Build history of the part. All positions in model axes, mm. A direction names the side the tool comes from. Round coordinates to 2 decimals unless told otherwise and drop trailing zeros. Write each loop counter-clockwise with the first axis right and the second up, starting at its lowest first coordinate (ties: lowest second). Pieces come first, ordered by that corner, then holes.
Item 1: 3-axis set-ups, long thin cutter, end or side, ignore diameter. For faces 1 (the flat face through (-23, 42.483, 3)), 2 (the flat face through (21.963, 47, 3)), 3 (the flat face through (37, 9.483, 3)): which of +Z, -Z, +X, -X, +Y, -Y reach the whole face in a straight line?
Item 2: Band-saw the part on B-B, the plane x = -21. Write the cut outline in (y, z), then the cut area to 3 significant figures.
Item 3: Wall check: probe 1 along X at (y, z) = (14.5, 2.5); probe 2 along Y at (x, z) = (2.5, 5); probe 3 along X at (y, z) = (-18, 0.5). Give the ranges that are in metal, low to high.
Item 4: Band-saw the part on D-D, the plane z = 2.5. Count the separate pieces of the cut face and the enclosed holes in it, then the cut area to 3 significant figures.
Item 5: Drop flat-ended pins along their axis: pin 1 Ø1.8 at (x, z) = (36.5, 2) entering from +Y; pin 2 Ø1 at (x, z) = (33, 2) entering from -Y; pin 3 Ø1.5 at (y, z) = (-8.5, 5.5) entering from +X. Give the stop position or say it passes through.
Item 6: Mould opens along Y. For faces 4 (the flat face through (27, -25.517, 3)), 5 (the cylindrical face through (21.393, 51.882, 3.131)), 6 (the cylindrical face through (7.86, 9.5, 3.22)) say: +Y half, -Y half, draft (parallel to the pull), parting line (faces both ways), or undercut.
Item 7: Band-saw the part on C-C, the plane y = -21. Write the cut outline in (x, z), then the cut area to 3 significant figures.
Item 8: Band-saw the part on A-A, the plane x = -5.5. Write the cut outline in (y, z).
```python
from build123d import *

# Parameters (mm, degrees)
EXTRUDE_1_DEPTH     = 6.35
SKETCH_2_R          = 1.5
CUT_EXTRUDE_1_DEPTH = 7.35
SKETCH_3_R          = 3
SKETCH_3_R_2        = 1.5
CUT_EXTRUDE_2_DEPTH = 7.35


with BuildPart() as part:
    # 草图1 → 凸台-拉伸1 (new body)
    with BuildSketch(Plane.XY):
        with BuildLine():
            Line((-28.036772487, 40.483201058), (-28.036772487, 21.483201058))
            ThreePointArc((-28.036772487, 21.483201058), (-28.622558924, 20.068987496), (-30.036772487, 19.483201058))
            Line((-30.036772487, 19.483201058), (-36.036772487, 19.483201058))
            ThreePointArc((-36.036772487, 19.483201058), (-37.450986049, 18.897414621), (-38.036772487, 17.483201058))
            Line((-38.036772487, 17.483201058), (-38.036772487, 11.483201058))
            ThreePointArc((-38.036772487, 11.483201058), (-37.450986049, 10.068987496), (-36.036772487, 9.483201058))
            Line((-36.036772487, 9.483201058), (-30.036772487, 9.483201058))
            ThreePointArc((-30.036772487, 9.483201058), (-28.622558924, 8.897414621), (-28.036772487, 7.483201058))
            Line((-28.036772487, 7.483201058), (-28.036772487, -23.516798942))
            ThreePointArc((-28.036772487, -23.516798942), (-27.450986049, -24.931012504), (-26.036772487, -25.516798942))
            Line((-26.036772487, -25.516798942), (-20.036772487, -25.516798942))
            ThreePointArc((-20.036772487, -25.516798942), (-18.622558924, -26.102585379), (-18.036772487, -27.516798942))
            Line((-18.036772487, -27.516798942), (-18.036772487, -33.516798942))
            ThreePointArc((-18.036772487, -33.516798942), (-17.450986049, -34.931012504), (-16.036772487, -35.516798942))
            Line((-16.036772487, -35.516798942), (19.963227513, -35.516798942))
            ThreePointArc((19.963227513, -35.516798942), (21.377441076, -34.931012504), (21.963227513, -33.516798942))
            Line((21.963227513, -33.516798942), (21.963227513, -27.516798942))
            ThreePointArc((21.963227513, -27.516798942), (22.549013951, -26.102585379), (23.963227513, -25.516798942))
            Line((23.963227513, -25.516798942), (29.963227513, -25.516798942))
            ThreePointArc((29.963227513, -25.516798942), (31.377441076, -24.931012504), (31.963227513, -23.516798942))
            Line((31.963227513, -23.516798942), (31.963227513, 7.483201058))
            ThreePointArc((31.963227513, 7.483201058), (32.549013951, 8.897414621), (33.963227513, 9.483201058))
            Line((33.963227513, 9.483201058), (39.963227513, 9.483201058))
            ThreePointArc((39.963227513, 9.483201058), (41.377441076, 10.068987496), (41.963227513, 11.483201058))
            Line((41.963227513, 11.483201058), (41.963227513, 17.483201058))
            ThreePointArc((41.963227513, 17.483201058), (41.377441076, 18.897414621), (39.963227513, 19.483201058))
            Line((39.963227513, 19.483201058), (33.963227513, 19.483201058))
            ThreePointArc((33.963227513, 19.483201058), (32.549013951, 20.068987496), (31.963227513, 21.483201058))
            Line((31.963227513, 21.483201058), (31.963227513, 40.483201058))
            ThreePointArc((31.963227513, 40.483201058), (31.377441076, 41.897414621), (29.963227513, 42.483201058))
            Line((29.963227513, 42.483201058), (23.963227513, 42.483201058))
            ThreePointArc((23.963227513, 42.483201058), (22.549013951, 43.068987496), (21.963227513, 44.483201058))
            Line((21.963227513, 44.483201058), (21.963227513, 50.483201058))
            ThreePointArc((21.963227513, 50.483201058), (21.377441076, 51.897414621), (19.963227513, 52.483201058))
            Line((19.963227513, 52.483201058), (-16.036772487, 52.483201058))
            ThreePointArc((-16.036772487, 52.483201058), (-17.450986049, 51.897414621), (-18.036772487, 50.483201058))
            Line((-18.036772487, 50.483201058), (-18.036772487, 44.483201058))
            ThreePointArc((-18.036772487, 44.483201058), (-18.622558924, 43.068987496), (-20.036772487, 42.483201058))
            Line((-20.036772487, 42.483201058), (-26.036772487, 42.483201058))
            ThreePointArc((-26.036772487, 42.483201058), (-27.450986049, 41.897414621), (-28.036772487, 40.483201058))
        make_face()
    extrude(amount=EXTRUDE_1_DEPTH)

    # 草图2 → 切除-拉伸1 (cut, through all)
    with BuildSketch(Plane.XY.offset(6.35)):
        with Locations((-33.036772487, 14.483201058)):
            Circle(SKETCH_2_R)
        with Locations((36.963227513, 14.483201058)):
            Circle(SKETCH_2_R)
    extrude(amount=-CUT_EXTRUDE_1_DEPTH, mode=Mode.SUBTRACT)

    # 草图3 → 切除-拉伸2 (cut, through all)
    with BuildSketch(Plane.XY.offset(6.35)):
        with Locations((1.963227513, 8.483201058)):
            Circle(SKETCH_3_R)
        with Locations((8.963227513, 8.483201058)):
            Circle(SKETCH_3_R_2)
        with Locations((1.963227513, 15.483201058)):
            Circle(SKETCH_3_R_2)
        with Locations((-5.036772487, 8.483201058)):
            Circle(SKETCH_3_R_2)
        with Locations((1.963227513, 1.483201058)):
            Circle(SKETCH_3_R_2)
    extrude(amount=-CUT_EXTRUDE_2_DEPTH, mode=Mode.SUBTRACT)


solid = part.part
```
Results:
1. face 1: +Z, -Z, -X, +Y
1. face 2: +Z, -Z, +X, +Y
1. face 3: +Z, -Z, +X, -Y
2. outline: (-25.52, 0) - (42.48, 0) - (42.48, 6.35) - (-25.52, 6.35) - close
2. area: 432 mm2
3. probe 1: x = -38.04 to -34.54, -31.54 to 0.83, 3.1 to 35.46, 38.46 to 41.96
3. probe 2: y = -35.52 to 0.08, 2.88 to 5.53, 11.43 to 14.08, 16.88 to 52.48
3. probe 3: x = -28.04 to 31.96
4. separate pieces: 1
4. enclosed holes: 7
4. area: 5,010 mm2
5. pin 1: stops at y = 19.48
5. pin 2: stops at y = 8.85
5. pin 3: stops at x = 31.96
6. face 4: -Y half
6. face 5: +Y half
6. face 6: undercut
7. outline: (-28.04, 0) - (31.96, 0) - (31.96, 6.35) - (-28.04, 6.35) - close
7. area: 381 mm2
8. outline: (-35.52, 0) - (7.06, 0) - (7.06, 6.35) - (-35.52, 6.35) - close; (9.91, 0) - (52.48, 0) - (52.48, 6.35) - (9.91, 6.35) - close
